Autodesk Inventor part; units mm, degrees
ref_plane "YZ Plane" through (0, 0, 0) normal (1, 0, 0) x (0, 1, 0)
ref_plane "XZ Plane" through (0, 0, 0) normal (0, 1, 0) x (-1, 0, 0)
ref_plane "XY Plane" through (0, 0, 0) normal (0, 0, 1) x (1, 0, 0)
sketch "Sketch1" plane through (0, 0, 0) normal (0, 0, 1) x (1, 0, 0)
  line L0 (-7.5, -26) -> (7.5, -26)
  line L1 (7.5, -26) -> (7.5, 26)
  line L2 (7.5, 26) -> (-7.5, 26)
  line L3 (-7.5, 26) -> (-7.5, -26)
  line L4 (-7.5, -26) -> (7.5, 26) construction
  line L5 (7.5, -26) -> (-7.5, 26) construction
  line L6 (0, 26) -> (0, 18)
  circle A0 centre (0, 18) radius 5.25
  line L7 (0, -26) -> (0, -22)
  line L8 (-3, -22) -> (3, -22)
  circle A1 centre (-3, -22) radius 1.5
  circle A2 centre (3, -22) radius 1.5
  point P0 (0, 0)
  dimension "d0" = 15
  dimension "d1" = 52
  dimension "d2" = 8
  dimension "d3" = 10.5
  dimension "d6" = 4
  dimension "d7" = 6
  dimension "d8" = 3
  dimension "d9" = 3
extrude "Extrusion1" add sketch "Sketch1" against normal blind 2
chamfer "Chamfer1" distance 2 angle 45 4 edges at (7.5, 26, -1) (-7.5, 26, -1) (7.5, -26, -1) (-7.5, -26, -1)
hole "Hole1" at (-3, -22, 0) at (3, -22, 0) direction (0, 0, -1) diameter 3.4 end through all
properties part number "Loadcell_lever"
CAD build for the part. Positions are in the model's coordinates, mm. Give positions to 0.01 mm unless a question says otherwise; leave off trailing zeros. Write each loop counter-clockwise with the first axis right and the second up, starting at its lowest first coordinate (ties: lowest second). Pieces come first, ordered by that corner, then holes. Notation, with made-up numbers: (-10.5, -12) -> (36.5, -12) arc R9 ccw to (36.5, -1) -> close; hole circle Ø3 at (25, 59). An arc over 180 degrees is marked (long way). Return JSON: item names as keys, results as strings.
Item 1: Two-plate mould, pull along Y, no slides. Class faces 1 (the flat face through (-6.5, 25, -1)), 2 (the cylindrical face through (2.42, 13.34, -0.99)), 3 (the flat face through (0, -26, -1)), 4 (the flat face through (-7.5, 0, -1)): +Y half, -Y half, draft (parallel to the pull), parting line (faces both ways), or undercut.
Answer below:
{"face 1": "+Y half", "face 2": "undercut", "face 3": "-Y half", "face 4": "draft"}
Item 2: Band-saw the part on A-A (x = 0). List the corners of the cut face in (y, z).
Answer below:
{"outline": "(-26, -2) -> (12.75, -2) -> (12.75, 0) -> (-26, 0) -> close; (23.25, -2) -> (26, -2) -> (26, 0) -> (23.25, 0) -> close"}
Item 3: Band-saw the part on D-D (z = -0.7). List the corners of the cut face in (x, y), then the cut area to 3 significant figures.
Answer below:
{"outline": "(-7.5, -24) -> (-5.5, -26) -> (5.5, -26) -> (7.5, -24) -> (7.5, 24) -> (5.5, 26) -> (-5.5, 26) -> (-7.5, 24) -> close; hole circle Ø10.5 at (0, 18); hole circle Ø3.4 at (-3, -22); hole circle Ø3.4 at (3, -22)", "area": "667 mm2"}
Item 4: Band-saw the part on B-B (y = 18). List the corners of the cut face in (x, z).
Answer below:
{"outline": "(-7.5, -2) -> (-5.25, -2) -> (-5.25, 0) -> (-7.5, 0) -> close; (5.25, -2) -> (7.5, -2) -> (7.5, 0) -> (5.25, 0) -> close"}
Item 5: Drill centre lines: probe 1 along X at (y, z) = (-22, -1.1); probe 2 along Y at (x, z) = (4, -0.2); probe 3 along X at (y, z) = (18, -0.45). Where is each one in solid material? Low to high.
Answer below:
{"probe 1": "x = -7.5 to -4.7, -1.3 to 1.3, 4.7 to 7.5", "probe 2": "y = -26 to -23.37, -20.63 to 14.6, 21.4 to 26", "probe 3": "x = -7.5 to -5.25, 5.25 to 7.5"}
Item 6: Band-saw the part on C-C (x = -3.5). List the corners of the cut face in (y, z), then the cut area to 3 significant figures.
Answer below:
{"outline": "(-26, -2) -> (-23.62, -2) -> (-23.62, 0) -> (-26, 0) -> close; (-20.38, -2) -> (14.09, -2) -> (14.09, 0) -> (-20.38, 0) -> close; (21.91, -2) -> (26, -2) -> (26, 0) -> (21.91, 0) -> close", "area": "81.8 mm2"}
